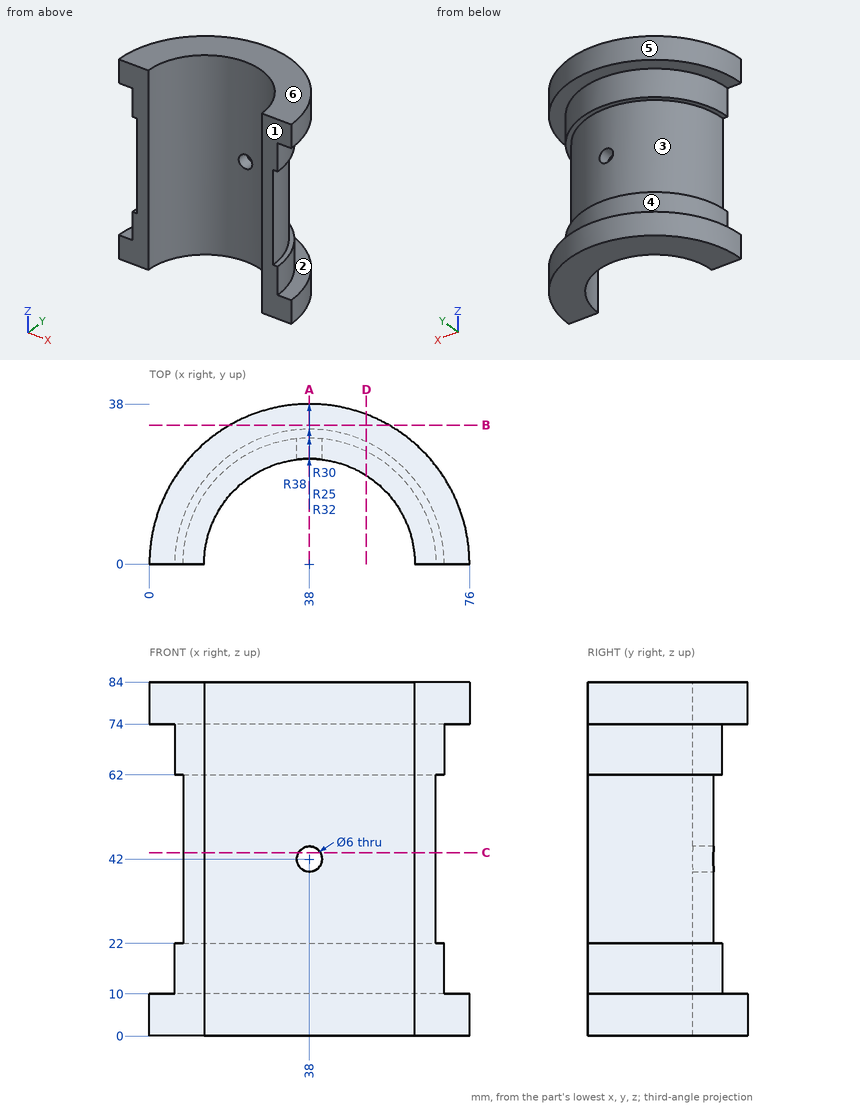
Source: three-view drawing plus pictorial views. Frame: mm from the lowest corner of the part. A direction names the side the tool comes from. Give positions to 0.01 mm unless a question says otherwise; leave off trailing zeros. Loops run counter-clockwise (first coordinate to the right, second up) from the corner with the lowest first, then second, coordinate; pieces in that order, holes last. Notation, with made-up numbers: (68.25, 10) -> (112.25, 10) arc R13 cw to (112.25, 35) -> close; hole circle Ø1 at (-14, 17.5). An arc over 180 degrees is marked (long way). Use a Markdown table: item, result. Add a question column.
(1) Ray query, line 1 (Z direction, x = 38, y = 27.8); line 2 (Z direction, x = 48, y = 28.5); line 3 (X direction, y = 10, z = 30). Return the intervals inside material, ascending.
(2) First-contact query: pin 1 Ø3.5 at (x, z) = (38, 42) entering from -Y; pin 2 Ø1.5 at (x, z) = (18.5, 18) entering from +Y; pin 3 Ø6 at (x, z) = (39.5, 37.5) entering from +Y; pin 4 Ø4 at (y, z) = (11, 65.5) entering from +X. Flat tips, straight axial feed; report the tip coordinate or a pass-through.
(3) Section query D-D (x = 51.5). Output: boundary loops of the cut face in (y, z), then the cut area to 3 significant figures.
(4) Section query A-A (x = 38). Output: boundary loops of the cut face in (y, z), then the cut area to 3 significant figures.
(5) Access query for the marked faces 1 and 2. Directions: +Z, -Z, +X, -X, +Y, -Y. A direction counts if a zero-diameter tool reaches every point of the face in a straight line with its end or side. Return the directions, or none.
(6) Section query C-C (z = 43.5). Output: boundary loops of the cut face in (x, y).
(7) Pull-direction query (Z, two-part tool) for the marked faces 3, 4, 5 and 6; classes: +Z half, -Z half, draft (parallel to the pull), parting line (faces both ways), or undercut.
(8) Section query B-B (y = 33). Output: boundary loops of the cut face in (x, z).
Checked values:
| question | item | result |
|---|---|---|
| 1 | line 1 | 0 to 39, 45 to 84 |
| 1 | line 2 | 0 to 22, 62 to 84 |
| 1 | line 3 | 9.72 to 15.09, 60.91 to 66.28 |
| 2 | pin 1 | through |
| 2 | pin 2 | y = 25.93 |
| 2 | pin 3 | y = 30 |
| 2 | pin 4 | x = 68.71 |
| 3 | outline | (21.04, 0) -> (35.52, 0) -> (35.52, 10) -> (29.01, 10) -> (29.01, 22) -> (26.79, 22) -> (26.79, 62) -> (29.01, 62) -> (29.01, 74) -> (35.52, 74) -> (35.52, 84) -> (21.04, 84) -> close |
| 3 | area | 711 mm^2 |
| 4 | outline | (25, 0) -> (38, 0) -> (38, 10) -> (32, 10) -> (32, 22) -> (30, 22) -> (30, 39) -> (25, 39) -> close; (25, 45) -> (30, 45) -> (30, 62) -> (32, 62) -> (32, 74) -> (38, 74) -> (38, 84) -> (25, 84) -> close |
| 4 | area | 598 mm^2 |
| 5 | face 1 | +Z, -Z, +X, -X, -Y |
| 5 | face 2 | +Y |
| 6 | outline | (8, 0) -> (13, 0) arc R25 cw to (35.4, 24.86) -> (35.4, 29.89) arc R30 ccw to start; (40.6, 24.86) arc R25 cw to (63, 0) -> (68, 0) arc R30 ccw to (40.6, 29.89) -> close |
| 7 | face 3 | undercut |
| 7 | face 4 | undercut |
| 7 | face 5 | draft |
| 7 | face 6 | +Z half |
| 8 | outline | (19.16, 0) -> (56.84, 0) -> (56.84, 10) -> (19.16, 10) -> close; (19.16, 74) -> (56.84, 74) -> (56.84, 84) -> (19.16, 84) -> close |
